Source: CAD feature listing. Evaluate the final solid. Frame: model axes, mm. Face numbers are marked on the shaded views. A direction names the side the tool comes from. Give positions to 0.01 mm unless a question says otherwise; leave off trailing zeros. Write each loop counter-clockwise with the first axis right and the second up, starting at its lowest first coordinate (ties: lowest second). Pieces come first, ordered by that corner, then holes. Notation, with made-up numbers: M 63.5,39 L 74.5,39 A14 cw 74.5,63 Z; hole C 23,-29.75 d3. An arc over 180 degrees is marked long. Return JSON: item names as keys, results as strings.
```python
from build123d import *

# Parameters (mm, degrees)
F1_DEPTH = 27
F2_W     = 5
F2_H     = 16
F3_DEPTH = 25
F4_W     = 10
F4_H     = 5
F5_DEPTH = 25


with BuildPart() as f1:
    # F0 (on Front) → F1 (new body)
    with BuildSketch(Plane.XZ):
        Polygon((0, 15.5563491861), (0, 0), (15.5563491861, 0), (13.7885822331, 1.767766953), (1.0606601718, 14.4956890143), align=None)
        Polygon((4.8765578995, 6.2907714619), (6.2907714619, 7.7049850243), (8.0585384149, 5.9372180713), (6.6443248525, 4.5230045089), align=None, mode=Mode.SUBTRACT)
        Polygon((3.5355339059, 19.091883092), (0, 15.5563491861), (1.0606601718, 14.4956890143), (4.5961940777, 18.0312229203), align=None)
        Polygon((13.7885822331, 1.767766953), (15.5563491861, 0), (19.091883092, 3.5355339059), (17.3241161391, 5.3033008589), align=None)
        Polygon((19.091883092, 3.5355339059), (15.5563491861, 0), (19.091883092, 0), align=None)
    extrude(amount=F1_DEPTH)

    # F2 (on face) → F3 (cut)
    with BuildSketch(Plane(origin=(-6.7175144213, 0, 6.7175144213), x_dir=(0.7071067812, 0, 0.7071067812), z_dir=(0.7071067812, 0, -0.7071067812))):
        with Locations((13.5, 13.5)):
            Rectangle(F2_W, F2_H)
    extrude(amount=-F3_DEPTH, mode=Mode.SUBTRACT)

    # F4 (on face) → F5 (cut)
    with BuildSketch(Plane(origin=(6.0104076401, 0, -6.0104076401), x_dir=(0, -1, 0), z_dir=(-0.7071067812, 0, 0.7071067812))):
        with Locations((13.5, 13.5)):
            Rectangle(F4_W, F4_H)
    extrude(amount=-F5_DEPTH, mode=Mode.SUBTRACT)


solid = f1.part
```
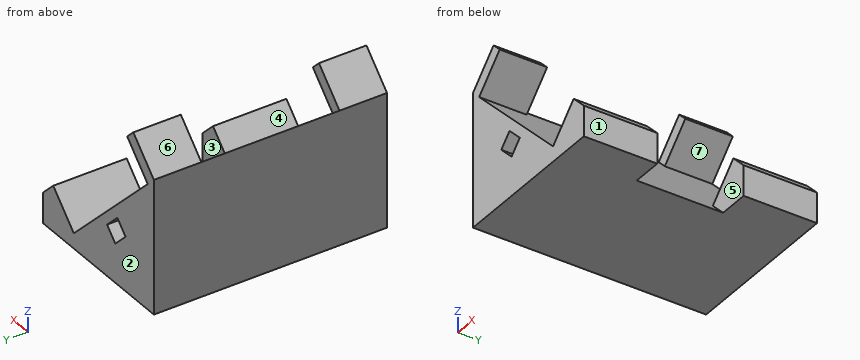
1) Contact query for flat-ended pins moving along their axis: pin 1 Ø6 at (x, z) = (12.5, 3.5) entering from +Y; pin 2 Ø5 at (x, y) = (10.5, -15) entering from +Z. Output: stop coordinate, or through.
Numbers:
{"pin 1": "stops at y = 0", "pin 2": "stops at z = 7.56"}
2) Cut plane C-C, the plane z = 16. Return the cut outline in (x, y), then the cut area to 3 significant figures.
Numbers:
{"outline": "M 0.44,-27 L 2.56,-27 L 2.56,-21.5 L 0.44,-21.5 Z; M 0.44,-5.5 L 2.56,-5.5 L 2.56,0 L 0.44,0 Z", "area": "23.3 mm²"}
3) Set-up query: the marked faces 4, 5, 6 and 7. Return all of +Z, -Z, +X, -X, +Y, -Y with unobstructed straight access to the full face (end or side cutting, diameter ignored); none if empty.
Numbers:
{"face 4": "+Z, +Y, -Y", "face 5": "+Z, +X", "face 6": "+Z, -X, +Y, -Y", "face 7": "+X, +Y, -Y"}
4) Cut plane D-D, the plane y = -4.25. Return the cut outline in (x, z), then the cut area to 3 significant figures.
Numbers:
{"outline": "M 0,0 L 19.09,0 L 19.09,3.54 L 17.32,5.3 L 13.79,1.77 L 1.06,14.5 L 4.6,18.03 L 3.54,19.09 L 0,15.56 Z; hole M 4.88,6.29 L 6.64,4.52 L 8.06,5.94 L 6.29,7.7 Z", "area": "142 mm²"}
5) Cut plane B-B, the plane x = 7. Return the cut outline in (y, z), then the cut area to 3 significant figures.
Numbers:
{"outline": "M -27,0 L 0,0 L 0,4.88 L -27,4.88 Z; M -27,7 L 0,7 L 0,8.56 L -27,8.56 Z", "area": "174 mm²"}
6) Draft query along Y for the marked faces 1, 2 and 3. Return one class per face: released by +Y, released by -Y, zero draft, split by the parting line, or undercut.
Numbers:
{"face 1": "zero draft", "face 2": "released by +Y", "face 3": "undercut"}
7) Line query: line 1 (Y direction, x = 3, z = 16.75); line 2 (Y direction, x = 16.25, z = 3); line 3 (Z direction, x = 1.75, y = -25.25). Output: solid intervals per line, ascending. Write a range as [from, to].
Numbers:
{"line 1": "y = [-27, -21.5], [-5.5, 0]", "line 2": "y = [-27, -18.5], [-8.5, 0]", "line 3": "z = [0, 13.81], [15.19, 17.31]"}
8) Cut plane A-A, the plane y = -19.5. Return the cut outline in (x, z).
Numbers:
{"outline": "M 0,0 L 19.09,0 L 19.09,3.54 L 17.32,5.3 L 13.79,1.77 L 0,15.56 Z; hole M 4.88,6.29 L 6.64,4.52 L 8.06,5.94 L 6.29,7.7 Z"}
